CAD build for the part. Positions are in the model's coordinates, mm. A direction names the side the tool comes from. Round coordinates to 2 decimals unless told otherwise and drop trailing zeros. Write each loop counter-clockwise with the first axis right and the second up, starting at its lowest first coordinate (ties: lowest second). Pieces come first, ordered by that corner, then holes. Notation, with made-up numbers: (0, 72.25) - (17, 72.25) arc R18 ccw to (17, 104.25) - close; hole circle Ø10 at (43.5, 48). An arc over 180 degrees is marked (long way). Answer in a Markdown table with one row per item.
```python
from build123d import *

# Parameters (mm, degrees)
SKETCH1_R           = 1.7
BOSS_EXTRUDE1_DEPTH = 3.8


with BuildPart() as part:
    # Sketch1 → Boss-Extrude1 (new body)
    with BuildSketch(Plane.XY):
        with BuildLine():
            Line((3.000019473, 70.3), (31.700019473, 70.3))
            ThreePointArc((31.700019473, 70.3), (33.114233035, 69.714213562), (33.700019473, 68.3))
            Line((33.700019473, 68.3), (33.700019473, 13.5))
            Line((33.700019473, 13.5), (37.350019473, 13.5))
            ThreePointArc((37.350019473, 13.5), (38.764233035, 12.914213562), (39.350019473, 11.5))
            Line((39.350019473, 11.5), (39.350019473, -11.641128199))
            ThreePointArc((39.350019473, -11.641128199), (38.764233035, -13.055341761), (37.350019473, -13.641128199))
            Line((37.350019473, -13.641128199), (31.700019473, -13.641128199))
            Line((31.700019473, -13.641128199), (3.000019473, -13.641128199))
            Line((3.000019473, -13.641128199), (-5.649980527, -13.641128199))
            ThreePointArc((-5.649980527, -13.641128199), (-7.064194089, -13.055341761), (-7.649980527, -11.641128199))
            Line((-7.649980527, -11.641128199), (-7.649980527, 11.5))
            ThreePointArc((-7.649980527, 11.5), (-7.064194089, 12.914213562), (-5.649980527, 13.5))
            Line((-5.649980527, 13.5), (1.000019473, 13.5))
            Line((1.000019473, 13.5), (1.000019473, 68.3))
            ThreePointArc((1.000019473, 68.3), (1.585805911, 69.714213562), (3.000019473, 70.3))
        make_face()
        with Locations(Location((11.15, 17.7, 0), (0, 0, 180))):
            Circle(SKETCH1_R, mode=Mode.SUBTRACT)
        with Locations(Location((9.85, 10, 0), (0, 0, 180))):
            Circle(SKETCH1_R, mode=Mode.SUBTRACT)
        with Locations(Location((24.85, 10, 0), (0, 0, 180))):
            Circle(SKETCH1_R, mode=Mode.SUBTRACT)
        with Locations(Location((9.85, -10, 0), (0, 0, 180))):
            Circle(SKETCH1_R, mode=Mode.SUBTRACT)
        with Locations(Location((24.85, -10, 0), (0, 0, 180))):
            Circle(SKETCH1_R, mode=Mode.SUBTRACT)
        with Locations(Location((23.55, 17.7, 0), (0, 0, 180))):
            Circle(SKETCH1_R, mode=Mode.SUBTRACT)
        with Locations(Location((23.55, 68.1, 0), (0, 0, 180))):
            Circle(SKETCH1_R, mode=Mode.SUBTRACT)
        with Locations(Location((11.15, 68.1, 0), (0, 0, 180))):
            Circle(SKETCH1_R, mode=Mode.SUBTRACT)
        with BuildLine():
            Line((7.35, 64.190811085), (27.35, 64.190811085))
            ThreePointArc((27.35, 64.190811085), (28.764213562, 63.605024648), (29.35, 62.190811085))
            Line((29.35, 62.190811085), (29.35, 23.654008347))
            ThreePointArc((29.35, 23.654008347), (28.764213562, 22.239794784), (27.35, 21.654008347))
            Line((27.35, 21.654008347), (7.35, 21.654008347))
            ThreePointArc((7.35, 21.654008347), (5.935786438, 22.239794784), (5.35, 23.654008347))
            Line((5.35, 23.654008347), (5.35, 62.190811085))
            ThreePointArc((5.35, 62.190811085), (5.935786438, 63.605024648), (7.35, 64.190811085))
        make_face(mode=Mode.SUBTRACT)
    extrude(amount=BOSS_EXTRUDE1_DEPTH)


solid = part.part
```
Q1. Flat gauge pins, fed straight in: pin 1 (1.9 mm diameter, centred on x = -1.5, z = 1, fed in from +Y); pin 2 (1.1 mm diameter, centred on y = 52.5, z = 1.5, fed in from +X). Where does each tip first touch, or does it go through?
Computed:
| item | result |
|---|---|
| pin 1 | stops at y = 13.5 |
| pin 2 | stops at x = 33.7 |
Q2. Drill centre lines: line 1 (X direction, y = 17.7, z = 1.75); line 2 (X direction, y = -10, z = 1.5); line 3 (Y direction, x = 9.85, z = 1.5). Where is each one in solid material? Low to high.
Computed:
| item | result |
|---|---|
| line 1 | x = 1 to 9.45, 12.85 to 21.85, 25.25 to 33.7 |
| line 2 | x = -7.65 to 8.15, 11.55 to 23.15, 26.55 to 39.35 |
| line 3 | y = -13.64 to -11.7, -8.3 to 8.3, 11.7 to 16.6, 18.8 to 21.65, 64.19 to 67, 69.2 to 70.3 |
Q3. Saw through at A-A on y = -10. List the corners of the cut face in (x, z).
Computed:
| item | result |
|---|---|
| outline | (-7.65, 0) - (8.15, 0) - (8.15, 3.8) - (-7.65, 3.8) - close; (11.55, 0) - (23.15, 0) - (23.15, 3.8) - (11.55, 3.8) - close; (26.55, 0) - (39.35, 0) - (39.35, 3.8) - (26.55, 3.8) - close |
Q4. Saw through at D-D on x = 18. List the corners of the cut face in (y, z), then the cut area to 3 significant figures.
Computed:
| item | result |
|---|---|
| outline | (-13.64, 0) - (21.65, 0) - (21.65, 3.8) - (-13.64, 3.8) - close; (64.19, 0) - (70.3, 0) - (70.3, 3.8) - (64.19, 3.8) - close |
| area | 157 mm2 |
Q5. 3-axis set-ups, long thin cutter, end or side, ignore diameter. For faces 5 (the flat face through (16, 20, 0)), 6 (the cylindrical face through (28.78, 22.255, 1.873)), 7 (the flat face through (33.7, 41, 2)): which of +Z, -Z, +X, -X, +Y, -Y reach the whole face in a straight line?
Computed:
| item | result |
|---|---|
| face 5 | -Z, +X, -X, +Y, -Y |
| face 6 | +Z, -Z |
| face 7 | +Z, -Z, +X, +Y |
Q6. Saw through at B-B on y = 40. List the corners of the cut face in (x, z).
Computed:
| item | result |
|---|---|
| outline | (1, 0) - (5.35, 0) - (5.35, 3.8) - (1, 3.8) - close; (29.35, 0) - (33.7, 0) - (33.7, 3.8) - (29.35, 3.8) - close |
Q7. Saw through at C-C on z = 1.75. Count the separate pieces of the cut face and the enclosed holes in it, then the cut area to 3 significant figures.
Computed:
| item | result |
|---|---|
| separate pieces | 1 |
| enclosed holes | 9 |
| area | 2,040 mm2 |
Q8. Pull direction X, two halves, no side cores. Call faces 1 (the flat face through (17, 64.191, 2)), 2 (the cylindrical face through (22, 17, 2)), 3 (the flat face through (39.35, 0, 2)), 4 (the flat face through (17, 70.3, 2)): released by +X, released by -X, zero draft, split by the parting line, or undercut.
Computed:
| item | result |
|---|---|
| face 1 | undercut |
| face 2 | undercut |
| face 3 | released by +X |
| face 4 | zero draft |
